Drawing for the job (mm, zero at the part's lowest x, y, z). Coordinates: 2 decimals unless noted, no trailing zeros. Write each loop counter-clockwise with the first axis right and the second up, starting at its lowest first coordinate (ties: lowest second). Pieces come first, ordered by that corner, then holes. Notation, with made-up numbers: (25.5, 28.5) - (49.5, 28.5) arc R16 ccw to (49.5, 42.5) - close; hole circle Ø1 at (67.5, 81.25). An arc over 180 degrees is marked (long way). Write each question's results on one line, items separated by ' | '.
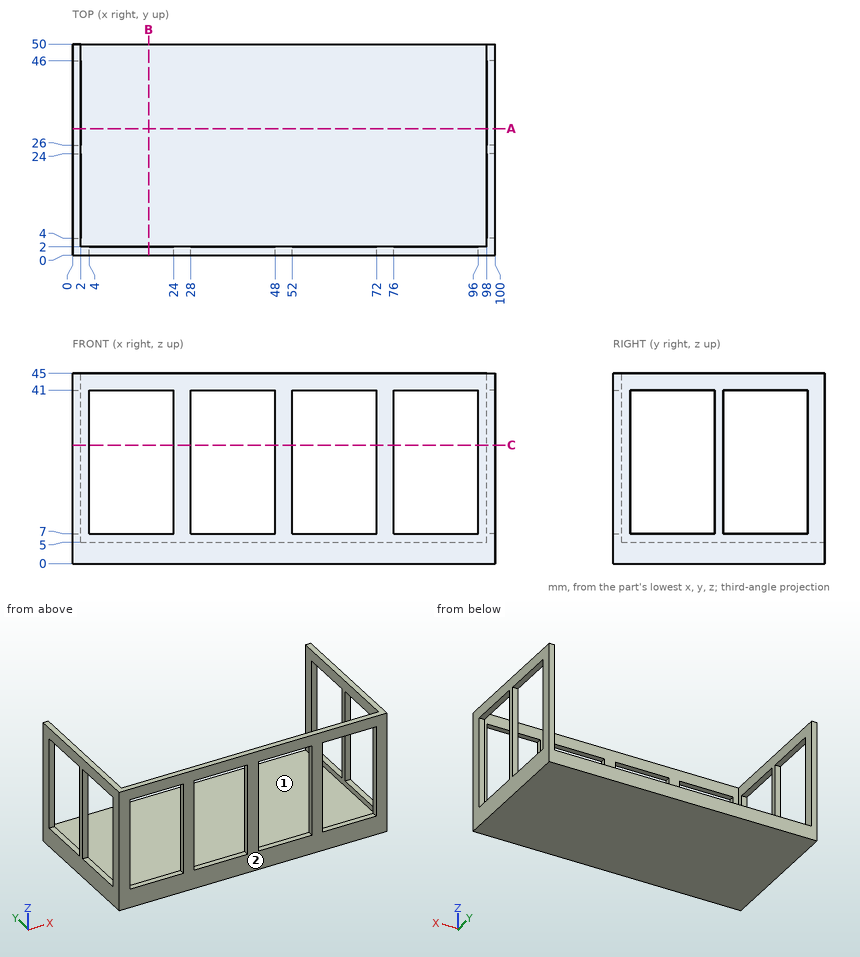
(1) Saw through at B-B on x = 18. Write the cut outline in (y, z).
Return value:
outline: (0, 0) - (50, 0) - (50, 5) - (2, 5) - (2, 7) - (0, 7) - close; (0, 41) - (2, 41) - (2, 45) - (0, 45) - close
(2) Two-plate mould, pull along X, no slides. Class the marked faces 1 and 2: released by +X, released by -X, zero draft, split by the parting line, or undercut.
Return value:
face 1: undercut | face 2: zero draft
(3) Wall check: line 1 (X direction, y = 6.5, z = 42.5); line 2 (Y direction, x = 50, z = 40); line 3 (Z direction, x = 59.5, y = 21). Give the ranges that are in metal, low to high. Write a range as from..to.
Return value:
line 1: x = 0..2, 98..100 | line 2: y = 0..2 | line 3: z = 0..5
(4) Saw through at A-A on y = 30. Write the cut outline in (x, z), then the cut area to 3 significant figures.
Return value:
outline: (0, 0) - (100, 0) - (100, 7) - (98, 7) - (98, 5) - (2, 5) - (2, 7) - (0, 7) - close; (0, 41) - (2, 41) - (2, 45) - (0, 45) - close; (98, 41) - (100, 41) - (100, 45) - (98, 45) - close | area: 524 mm^2
(5) Saw through at C-C on z = 28. Count the separate pieces of the cut face and the enclosed holes in it, then the cut area to 3 significant figures.
Return value:
separate pieces: 9 | enclosed holes: 0 | area: 72.0 mm^2
(6) Flat gauge pins, fed straight in: P1, Ø12, axis at x = 32, z = 27, coming from the +Y side; P2, Ø1.5, axis at x = 22.5, z = 31, coming from the +Y side. Where does each tip first touch, or does it go through?
Return value:
P1: stops at y = 2 | P2: passes through
